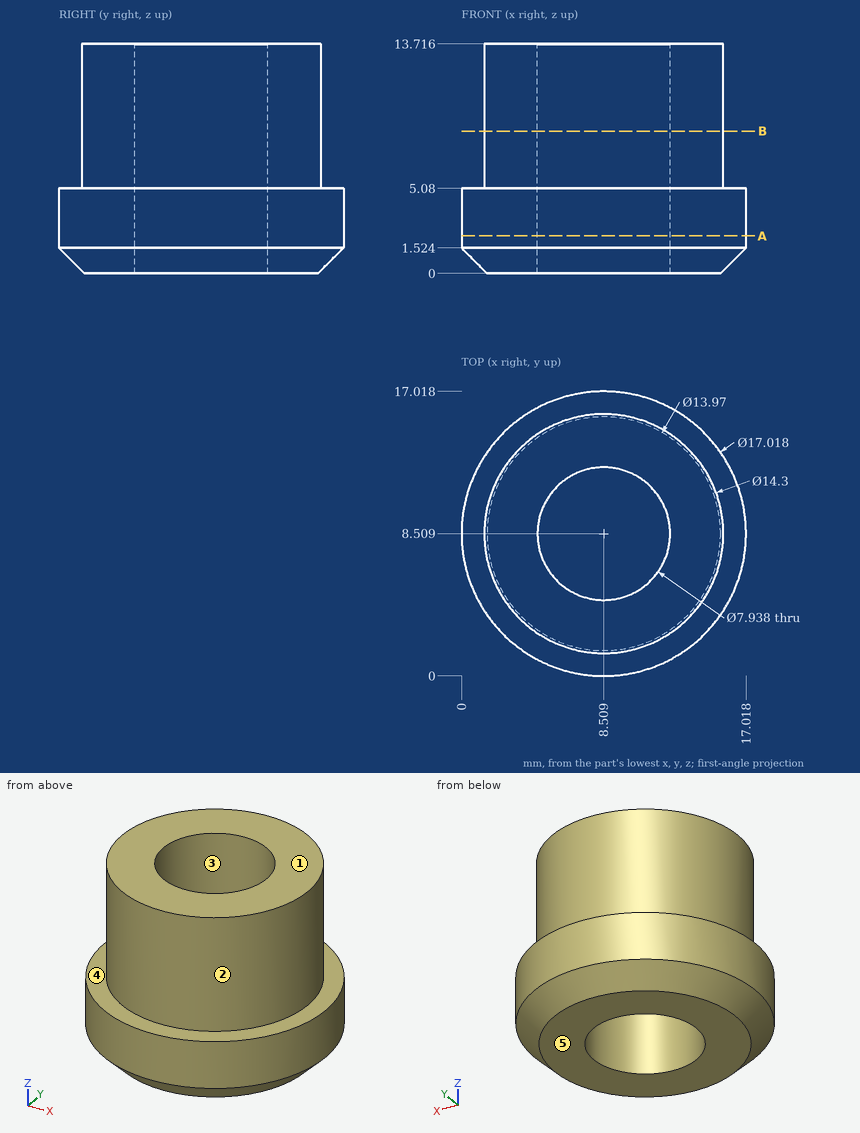
Job drawing, mm, ordinate dimensions from the low corner. One solid piece. A direction names the side the tool comes from. Give positions to 0.01 mm unless a question says otherwise; leave off trailing zeros. Loops run counter-clockwise (first coordinate to the right, second up) from the corner with the lowest first, then second, coordinate; pieces in that order, holes last.
Item 1: Slice it at A-A, the plane z = 2.25. List the corners of the cut face in (x, y).
Answers follow:
outline: circle Ø17.02 at (8.51, 8.51); hole circle Ø7.94 at (8.51, 8.51)
Item 2: Slice it at B-B, the plane z = 8.5. List the corners of the cut face in (x, y), and give its area (3 significant figures).
Answers follow:
outline: circle Ø14.3 at (8.51, 8.51); hole circle Ø7.94 at (8.51, 8.51)
area: 111 mm2
Item 3: Flat gauge pins, fed straight in: pin 1 (1 mm diameter, centred on x = 10, z = 4, fed in from -Y); pin 2 (1 mm diameter, centred on y = 10, z = 11.5, fed in from -X); pin 3 (7 mm diameter, centred on x = 8.509, y = 8.509, fed in from +Z). Where does each tip first touch, or does it go through?
Answers follow:
pin 1: stops at y = 0.06
pin 2: stops at x = 1.43
pin 3: passes through
Item 4: Drill centre lines: line 1 (X direction, y = 8.5, z = 11.25); line 2 (X direction, y = 10.75, z = 5.75) (1 decimal); line 3 (Y direction, x = 8, z = 8) (1 decimal). Where is each one in solid material? Low to high.
Answers follow:
line 1: x = 1.36 to 4.54, 12.48 to 15.66
line 2: x = 1.7 to 5.2, 11.8 to 15.3
line 3: y = 1.4 to 4.6, 12.4 to 15.6
Item 5: Pull direction X, two halves, no side cores. Call the marked faces 1, 2 and 3: released by +X, released by -X, zero draft, split by the parting line, or undercut.
Answers follow:
face 1: zero draft
face 2: split by the parting line
face 3: undercut
Item 6: Which spindle directions (+Z, -Z, +X, -X, +Y, -Y) get a long thin tool onto all of the face, cutting with end or side? Do the marked faces 4 and 5. Say none if no direction does.
Answers follow:
face 4: +Z
face 5: -Z, +X, -X, +Y, -Y
